```python
from build123d import *

# Parameters (mm, degrees)
F1_DEPTH = 63.5
F2_DEPTH = 25.4
F0_W     = 31.6445648432
F0_H     = 28.575
F3_DEPTH = 7.9375
F5_R     = 6.35


with BuildPart() as f1:
    # F0 (on Front) → F1 (new body, symmetric)
    with BuildSketch(Plane.XZ):
        Polygon((-41.275, -9.525), (41.275, -9.525), (41.275, 9.525), (22.225, 9.525), (-41.275, 9.525), align=None)
    extrude(amount=F1_DEPTH, both=True)

    # F0 (on Front) → F2 (join, symmetric)
    with BuildSketch(Plane.XZ):
        with BuildLine():
            Line((22.225, 9.525), (41.275, 9.525))
            Line((41.275, 9.525), (41.275, 25.1988060772))
            ThreePointArc((41.275, 25.1988060772), (45.9246798487, 36.4241262286), (57.15, 41.0738060772))
            Line((57.15, 41.0738060772), (66.675, 41.0738060772))
            Line((66.675, 41.0738060772), (66.675, 60.1238060772))
            Line((66.675, 60.1238060772), (57.15, 60.1238060772))
            add(Edge.make_bspline(
                [(56.3607333992, 60.1148866596), (56.6244550053, 60.118607245), (56.8875501507, 60.1215808142), (57.15, 60.1238060772)],
                knots=[109.9586728318, 109.9586728318, 109.9586728318, 109.9586728318, 110.6694167394, 110.6694167394, 110.6694167394, 110.6694167394], degree=3))
            ThreePointArc((56.3607333992, 60.1148866596), (32.1768067617, 49.6138679138), (22.225, 25.1988060772))
            Line((22.225, 25.1988060772), (22.225, 9.525))
        make_face()
    extrude(amount=F2_DEPTH, both=True)

    # F0 (on Front) → F3 (join, symmetric)
    with BuildSketch(Plane.XZ):
        Polygon((-41.275, -9.525), (41.275, -9.525), (41.275, 9.525), (22.225, 9.525), (-41.275, 9.525), align=None)
        with BuildLine():
            Line((22.225, 9.525), (41.275, 9.525))
            Line((41.275, 9.525), (41.275, 25.1988060772))
            ThreePointArc((41.275, 25.1988060772), (45.9246798487, 36.4241262286), (57.15, 41.0738060772))
            Line((57.15, 41.0738060772), (66.675, 41.0738060772))
            Line((66.675, 41.0738060772), (66.675, 60.1238060772))
            Line((66.675, 60.1238060772), (57.15, 60.1238060772))
            add(Edge.make_bspline(
                [(56.3607333992, 60.1148866596), (56.6244550053, 60.118607245), (56.8875501507, 60.1215808142), (57.15, 60.1238060772)],
                knots=[109.9586728318, 109.9586728318, 109.9586728318, 109.9586728318, 110.6694167394, 110.6694167394, 110.6694167394, 110.6694167394], degree=3))
            ThreePointArc((56.3607333992, 60.1148866596), (32.1768067617, 49.6138679138), (22.225, 25.1988060772))
            Line((22.225, 25.1988060772), (22.225, 9.525))
        make_face()
        with BuildLine():
            add(Edge.make_bspline(
                [(-41.275, 9.525), (-40.2339300381, 41.0838661131), (15.5605556063, 59.539277601), (56.3607333992, 60.1148866596)],
                knots=[0, 0, 0, 0, 109.9586728318, 109.9586728318, 109.9586728318, 109.9586728318], degree=3))
            Line((-41.275, 9.525), (22.225, 9.525))
            Line((22.225, 9.525), (22.225, 25.1988060772))
            ThreePointArc((22.225, 25.1988060772), (32.1768067617, 49.6138679138), (56.3607333992, 60.1148866596))
        make_face()
        with BuildLine():
            ThreePointArc((57.15, 60.1238060772), (56.7553415011, 60.1215761516), (56.3607333992, 60.1148866596))
            add(Edge.make_bspline(
                [(56.3607333992, 60.1148866596), (56.6244550053, 60.118607245), (56.8875501507, 60.1215808142), (57.15, 60.1238060772)],
                knots=[109.9586728318, 109.9586728318, 109.9586728318, 109.9586728318, 110.6694167394, 110.6694167394, 110.6694167394, 110.6694167394], degree=3))
        make_face()
        Polygon((66.675, 60.1238060772), (66.675, 41.0738060772), (66.675, 38.1), (85.8304351568, 38.1), (85.8304351568, 66.675), (66.675, 66.675), align=None)
        with Locations((101.6527175784, 52.3875)):
            Rectangle(F0_W, F0_H)
    extrude(amount=F3_DEPTH, both=True)

    # F0 (on Front) → F4 (revolve)
    with BuildSketch(Plane.XZ):
        with Locations((101.6527175784, 52.3875)):
            Rectangle(F0_W, F0_H)
    revolve(axis=Axis((85.8304351568, 0, 52.3875), (0, 0, 1)))

    # F5
    f5_edges = [f1.edges().sort_by_distance(p)[0] for p in [
        (-41.275, -63.5, 0),
        (41.275, -63.5, 0),
        (41.275, 63.5, 0),
        (-41.275, 63.5, 0),
    ]]
    fillet(f5_edges, radius=F5_R)


solid = f1.part
```
Source: CAD feature listing. Evaluate the final solid. Frame: model axes, mm. A direction names the side the tool comes from. Round coordinates to 2 decimals unless told otherwise and drop trailing zeros. Loops run counter-clockwise (first coordinate to the right, second up) from the corner with the lowest first, then second, coordinate; pieces in that order, holes last. Notation, with made-up numbers: M 87.25,18.5 L 93.25,18.5 A29 cw 93.25,54.5 Z; hole C 24,9.5 d8. An arc over 180 degrees is marked long. Use a Markdown table: item, result. Add a question column.
1. Set-up query: faces 4 (the flat face through (22.225, -17, 17)), 5 (the flat face through (60, 22, 60.124)), 6 (the flat face through (85, 0, 38.1)). Return all of +Z, -Z, +X, -X, +Y, -Y with unobstructed straight access to the full face (end or side cutting, diameter ignored); none if empty.
2. Cut plane A-A, the plane y = -53. Output: boundary loops of the cut face in (x, z) (3 decimals), and give its area (3 significant figures).
3. Pull-direction query (X, two-part tool) for faces 1 (the flat face through (60, -22, 60.124)), 2 (the flat face through (60, 22, 41.074)), 3 (the flat face through (-41.275, -1, 0)); classes: +X half, -X half, draft (parallel to the pull), parting line (faces both ways), or undercut.
4. Ray query, line 1 along X through (y, z) = (50, 7.5) (3 decimals); line 2 along Z through (x, y) = (-24.5, -16.5) (3 decimals); line 3 along Y through (x, z) = (41, 55). Return the intervals inside material, ascending. Write a range as [from, to].
5. Contact query for flat-ended pins moving along their axis: pin 1 (10.5 mm diameter, centred on x = 64, y = 17.5, fed in from -Z); pin 2 (10 mm diameter, centred on y = 39.5, z = 37, fed in from +X); pin 3 (17 mm diameter, centred on y = 18.5, z = 18.5, fed in from -X) (3 decimals); pin 4 (0.5 mm diameter, centred on x = 117, z = 58, fed in from -Y). Output: stop coordinate, or through.
Solution:
| question | item | result |
|---|---|---|
| 1 | face 4 | +Z, -X, -Y |
| 1 | face 5 | +Z, -X, +Y |
| 1 | face 6 | -Z, +X, +Y, -Y |
| 2 | outline | M -41.275,-9.525 L 41.275,-9.525 L 41.275,9.525 L -41.275,9.525 Z |
| 2 | area | 1,570 mm2 |
| 3 | face 1 | draft |
| 3 | face 2 | undercut |
| 3 | face 3 | -X half |
| 4 | line 1 | x = [-41.275, 41.275] |
| 4 | line 2 | z = [-9.525, 9.525] |
| 4 | line 3 | y = [-25.4, 25.4] |
| 5 | pin 1 | stops at z = 38.1 |
| 5 | pin 2 | passes through |
| 5 | pin 3 | stops at x = 22.225 |
| 5 | pin 4 | stops at y = -7.94 |
